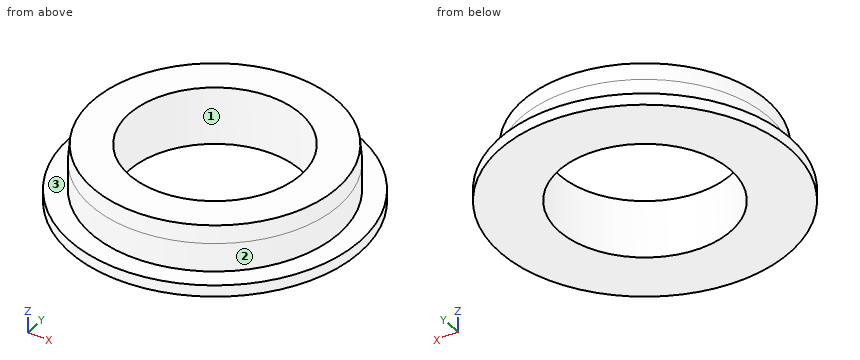
```python
from build123d import *

# Parameters (mm, degrees)
SKETCH1_R           = 24.13
BOSS_EXTRUDE1_DEPTH = 0.9525
SKETCH2_R           = 20.6375
BOSS_EXTRUDE2_DEPTH = 7.62
SKETCH4_R           = 14.2875
CUT_EXTRUDE1_DEPTH  = 10.525
CHAMFER1_SIZE       = 0.254
CHAMFER1_SIZE2      = 2.903233285


with BuildPart() as part:
    # Sketch1 → Boss-Extrude1 (new body, symmetric)
    with BuildSketch(Plane.XY):
        Circle(SKETCH1_R)
    extrude(amount=BOSS_EXTRUDE1_DEPTH, both=True)

    # Sketch2 → Boss-Extrude2 (add)
    with BuildSketch(Plane.XY.offset(0.9525)):
        Circle(SKETCH2_R)
    extrude(amount=BOSS_EXTRUDE2_DEPTH)

    # Sketch4 → Cut-Extrude1 (cut, through all)
    with BuildSketch(Plane(origin=(0, 0, -0.9525), x_dir=(-1, 0, 0), z_dir=(0, 0, -1))):
        Circle(SKETCH4_R)
    extrude(amount=-CUT_EXTRUDE1_DEPTH, mode=Mode.SUBTRACT)

    # Chamfer1
    chamfer1_edges = [part.edges().sort_by_distance(p)[0] for p in [
        (-20.6375, 0, 8.5725),
    ]]
    chamfer1_side = [part.faces().sort_by_distance(p)[0] for p in [
        (-20.053783352, 0, 8.5725),
    ]]
    chamfer(chamfer1_edges, length=CHAMFER1_SIZE, length2=CHAMFER1_SIZE2, reference=chamfer1_side[0])


solid = part.part
```
Input: part model. Units: mm. Frame: model coordinates. Face numbers are marked on the shaded views. Round coordinates to 2 decimals unless told otherwise and drop trailing zeros. Write each loop counter-clockwise with the first axis right and the second up, starting at its lowest first coordinate (ties: lowest second). Pieces come first, ordered by that corner, then holes. Notation, with made-up numbers: (-10, 82.5) -> (42, 82.5) arc R36 cw to (42, 116.5) -> close; hole circle Ø8 at (9, 76.5). An arc over 180 degrees is marked (long way). Answer as CSV lines item,"result".
1. Section C-C (z = 3). Return the cut outline in (x, y) (1 decimal).
Geometry says:
outline,"circle Ø41.3 at (0, 0); hole circle Ø28.6 at (0, 0)"
2. Contact query for flat-ended pins moving along their axis: P1, Ø1, axis at x = 0.5, z = 3.5, coming from the +Y side; P2, Ø3, axis at y = -19, z = 5, coming from the -X side; P3, Ø4, axis at x = 15, z = 2, coming from the +Y side. Output: stop coordinate, or through.
Geometry says:
P1,"stops at y = 20.64"
P2,"stops at x = -10.94"
P3,"stops at y = 20.14"
3. Section D-D (x = 21.5). Return the cut outline in (y, z).
Geometry says:
outline,"(-10.95, -0.95) -> (10.95, -0.95) -> (10.95, 0.95) -> (-10.95, 0.95) -> close"
4. Ray query, L1, parallel to Y at x = 0, z = 4; L2, parallel to Y at x = -10.5, z = 0.5; L3, parallel to X at y = 3, z = 4.75. Return the intervals inside material, ascending. Write a range as [from, to].
Geometry says:
L1,"y = [-20.64, -14.29], [14.29, 20.64]"
L2,"y = [-21.73, -9.69], [9.69, 21.73]"
L3,"x = [-20.42, -13.97], [13.97, 20.42]"
5. Section A-A (y = 0). Return the cut outline in (x, z).
Geometry says:
outline,"(-24.13, -0.95) -> (-14.29, -0.95) -> (-14.29, 8.57) -> (-20.38, 8.57) -> (-20.64, 5.67) -> (-20.64, 0.95) -> (-24.13, 0.95) -> close; (14.29, -0.95) -> (24.13, -0.95) -> (24.13, 0.95) -> (20.64, 0.95) -> (20.64, 5.67) -> (20.38, 8.57) -> (14.29, 8.57) -> close"
6. Mould query, pull axis Y, two halves, no side actions, for the marked faces 1, 2 and 3. Classes: +Y half, -Y half, draft (parallel to the pull), parting line (faces both ways), or undercut.
Geometry says:
face 1,"undercut"
face 2,"parting line"
face 3,"draft"
